Source: CAD feature listing. Evaluate the final solid. Frame: model axes, mm. A direction names the side the tool comes from. Coordinates: 2 decimals unless noted, no trailing zeros. Order: outer loops, then holes, each group sorted by start corner. A loop starts at its lowest first (then second) coordinate and runs counter-clockwise, first axis right, second up. Notation, with made-up numbers: (-31, 43) -> (0, 43) arc R8 cw to (0, 58) -> close; hole circle Ø5 at (12, 56). An arc over 180 degrees is marked (long way). Put each result on its own line as item: value.
Solid Edge part; units mm, degrees
sketch "Sketch1" plane through (0, 0, 0) normal (0, 0, 1) x (1, 0, 0)
  circle A0 centre (0, 0) radius 8
extrude "Protrusion1" add sketch "Sketch1" along normal blind 10
sketch "Sketch2" plane through (0, 0, 0) normal (0, 0, -1) x (1, 0, 0)
  circle A0 centre (0, 0) radius 5
extrude "Protrusion2" add sketch "Sketch2" along normal blind 60
sketch "Sketch3" plane through (0, 0, -60) normal (0, 0, -1) x (1, 0, 0)
  circle A0 centre (0, 0) radius 4.9997
extrude "Cutout1" cut sketch "Sketch3" against normal blind 32 flip side to cut
chamfer "Chamfer_1" distance 0.75 angle 45 1 edges at (-4.9997, 0, -60)
sketch "Sketch4" plane through (0, 0, 10) normal (0, 0, 1) x (1, 0, 0)
  line L0 (-2.3094, 4) -> (2.3094, 4)
  line L1 (4.6188, 0) -> (2.3094, 4)
  line L2 (2.3094, -4) -> (4.6188, 0)
  line L3 (-2.3094, -4) -> (2.3094, -4)
  line L4 (-4.6188, 0) -> (-2.3094, -4)
  line L5 (-2.3094, 4) -> (-4.6188, 0)
extrude "Cutout2" cut sketch "Sketch4" against normal blind 5
properties part number "24104593"
1. Pull-direction query (X, two-part tool) for faces 1 (the cylindrical face through (-1.08, -4.88, -13.8)), 2 (the flat face through (0, 0, -60)), 3 (the flat face through (-3.448, 2.028, 7.535)), 4 (the flat face through (3.48, 1.97, 7.54)); classes: pulls with the +X half, pulls with the -X half, needs draft (parallel to the pull), parting line crosses it, or undercut.
Numbers:
face 1: parting line crosses it
face 2: needs draft
face 3: undercut
face 4: undercut
2. Set-up query: faces 5 (the flat face through (0, 0, 5)), 6 (the cylindrical face through (-1.73, 7.81, 4.93)), 7 (the cylindrical face through (4.77, -1.5, -43.84)). Return all of +Z, -Z, +X, -X, +Y, -Y with unobstructed straight access to the full face (end or side cutting, diameter ignored); none if empty.
Numbers:
face 5: +Z
face 6: +Z, -Z
face 7: -Z
3. Cut plane C-C on y = -6.5. Output: boundary loops of the cut face in (x, z).
Numbers:
outline: (-4.66, 0) -> (4.66, 0) -> (4.66, 10) -> (-4.66, 10) -> close
4. Ray query, line 1 along Z through (x, y) = (-3, -1.25); line 2 along Z through (x, y) = (-5.5, -0.75); line 3 along X through (y, z) = (0.25, -17.5). Return the intervals inside material, ascending.
Numbers:
line 1: z = -60 to 5
line 2: z = 0 to 10
line 3: x = -4.99 to 4.99
5. Cut plane B-B on z = -54. Output: boundary loops of the cut face in (x, y), plus the area to 3 significant figures.
Numbers:
outline: circle Ø10 at (0, 0)
area: 78.5 mm2
6. First-contact query: pin 1 (1 mm diameter, centred on y = -5, z = -50.5, fed in from -X); pin 2 (1 mm diameter, centred on x = -3, y = 6.5, fed in from -Z); pin 3 (3.5 mm diameter, centred on x = -1, z = 8, fed in from +Y); pin 4 (5 mm diameter, centred on y = 6, z = -32, fed in from +X). Flat tips, straight axial feed; report the tip coordinate or a pass-through.
Numbers:
pin 1: stops at x = -2.18
pin 2: stops at z = 0
pin 3: stops at y = 8
pin 4: stops at x = 3.57
